```python
from build123d import *

# Parameters (mm, degrees)
F0_R            = 2.7
F1_DEPTH        = 8
F2_R            = 1.5
F3_DEPTH        = 11
F3_COPIES_COUNT = 3


# Not quite as in the source:
# - a pattern or mirror of a feature is missing from the dataset's text; its kind, count and spacing are read off the source's solid


with BuildPart() as f1:
    # F0 (on Top) → F1 (new body)
    with BuildSketch(Plane.XY):
        Polygon((30.9826352704, 105.0418671526), (-39.0173647296, 105.0418671526), (-59.0173647296, 70.4008510012), (-24.0173647296, 9.7790727363), (15.9826352704, 9.7790727363), (50.9826352704, 70.4008510012), align=None)
        with Locations((-4.0173647296, 41.7405969634)):
            Circle(F0_R, mode=Mode.SUBTRACT)
        Polygon((-14.0173647296, 19.7790727363), (-18.2438620377, 19.7790727363), (-47.4703593458, 70.4008510012), (-33.2438620377, 95.0418671526), (-14.0173647296, 95.0418671526), align=None, mode=Mode.SUBTRACT)
        Polygon((25.2091325785, 95.0418671526), (39.4356298866, 70.4008510012), (10.2091325785, 19.7790727363), (5.9826352704, 19.7790727363), (5.9826352704, 95.0418671526), align=None, mode=Mode.SUBTRACT)
        with Locations((-4.0173647296, 61.7405969634)):
            Circle(F0_R, mode=Mode.SUBTRACT)
        with Locations((-4.0173647296, 81.7405969634)):
            Circle(F0_R, mode=Mode.SUBTRACT)
    extrude(amount=F1_DEPTH)

    # F2 (on face) → F3 (cut)
    with BuildSketch(Plane.XZ.offset(-9.7790727363)):
        with Locations((10.9826352704, 4)):
            Circle(F2_R)
        with Locations((-19.0173647296, 4)):
            Circle(F2_R)
    f3 = extrude(amount=-F3_DEPTH, mode=Mode.SUBTRACT)

    # F3_copies: F3 ×3 about axis
    f3_copies_axis = Axis((-4.017365, 61.740597, 0), (0, 0, 1))
    for i in range(1, F3_COPIES_COUNT):
        add(f3.rotate(f3_copies_axis, i * 360 / F3_COPIES_COUNT), mode=Mode.SUBTRACT)


solid = f1.part
```
Here's how the part is built. I have some questions about the finished solid (model axes, mm). A direction names the side the tool comes from. Round coordinates to 2 decimals unless told otherwise and drop trailing zeros. Order: outer loops, then holes, each group sorted by start corner. A loop starts at its lowest first (then second) coordinate and runs counter-clockwise, first axis right, second up. Notation, with made-up numbers: M 77.25,70.5 L 134.25,70.5 A20 cw 134.25,107.5 Z; hole C 63,41.25 d9. An arc over 180 degrees is marked long. Answer in a Markdown table with one row per item.
Item 1: If I drill on L1, parallel to Y at x = -4, z = 1.5; L2, parallel to X at y = 80, z = 3; L3, parallel to X at y = 59, z = 3.5, over which ranges is the centre line in solid material (lowest first)? Write a range as from..to.
A:
| item | result |
|---|---|
| L1 | y = 9.78..39.04, 44.44..59.04, 64.44..79.04, 84.44..105.04 |
| L2 | x = -53.48..-41.93, -14.02..-6.08, -1.95..5.98, 33.89..45.44 |
| L3 | x = -52.44..-40.89, -14.02..5.98, 32.85..44.4 |
Item 2: Imagine slicing it at A-A, the plane x = -45.5. Write out the boundary of the cut face in (y, z), and give its area (3 significant figures).
A:
| item | result |
|---|---|
| outline | M 46.99,0 L 66.99,0 L 66.99,8 L 46.99,8 Z; M 73.81,0 L 93.81,0 L 93.81,8 L 73.81,8 Z |
| area | 320 mm2 |
Item 3: Imagine slicing it at D-D, the plane x = -27. Write out the boundary of the cut face in (y, z).
A:
| item | result |
|---|---|
| outline | M 14.95,0 L 34.95,0 L 34.95,8 L 14.95,8 Z; M 95.04,0 L 105.04,0 L 105.04,8 L 95.04,8 Z |
Item 4: Thinking about a two-plate mould opening in X: for faces 1 (the face through (-41.76, 40.51, 3.94)), 2 (the face through (15, 95.042, 4)), 3 (the face through (-4, 9.779, 4)), which applies, +X half, -X half, draft (parallel to the pull), parting line (faces both ways), or undercut?
A:
| item | result |
|---|---|
| face 1 | -X half |
| face 2 | undercut |
| face 3 | draft |
Item 5: Imagine slicing it at B-B, the plane z = 4. State how many separate pieces and enclosed holes the cut face has, and give its area (3 significant figures).
A:
| item | result |
|---|---|
| separate pieces | 5 |
| enclosed holes | 3 |
| area | 4,200 mm2 |
Item 6: Imagine slicing it at C-C, the plane y = 29. Write out the boundary of the cut face in (x, z), and give its area (3 significant figures).
A:
| item | result |
|---|---|
| outline | M -35.11,0 L -23.57,0 L -23.57,8 L -35.11,8 Z; M -14.02,0 L 5.98,0 L 5.98,8 L -14.02,8 Z; M 15.53,0 L 27.08,0 L 27.08,8 L 15.53,8 Z |
| area | 345 mm2 |
Item 7: For faces 4 (the face through (33.24, 39.67, 3.94)), 5 (the face through (25, 45.4, 3.9)), 6 (the face through (-20.516, 15.202, 4.066)), which set-ups out of +Z, -Z, +X, -X, +Y, -Y let a thin tool reach every point of the face, with its end or its side?
A:
| item | result |
|---|---|
| face 4 | +Z, -Z, +X, -Y |
| face 5 | +Z, -Z |
| face 6 | -Y |
Item 8: I'm going to push flat-ended pins straight in: pin 1 (3 mm diameter, centred on y = 55.5, z = 1, fed in from -X); pin 2 (4 mm diameter, centred on x = -28, z = 6, fed in from -Y); pin 3 (3 mm diameter, centred on x = 22.5, z = 3, fed in from -Y). Where does each tip first touch, or does it pass through?
A:
| item | result |
|---|---|
| pin 1 | stops at x = -51.28 |
| pin 2 | stops at y = 13.21 |
| pin 3 | stops at y = 18.47 |
